```python
from build123d import *

# Parameters (mm, degrees)
BOSS_EXTRUDE1_DEPTH = 13.2
CUT_EXTRUDE1_DEPTH  = 2.2
CUT_EXTRUDE5_DEPTH  = 3.2
CUT_EXTRUDE7_DEPTH  = 47.2


with BuildPart() as part:
    # Sketch1 → Boss-Extrude1 (new body)
    with BuildSketch(Plane(origin=(0, 0, 0), x_dir=(0, 0, -1), z_dir=(1, 0, 0))):
        Polygon((0, 0), (30.22758915, 0), (55.09957656, 33.798540965), (41.306638332, 146.917141225), (-10.793062749, 146.917141225), (-25.237530543, 33.798540965), align=None)
    extrude(amount=BOSS_EXTRUDE1_DEPTH)

    # Sketch2 → Cut-Extrude1 (cut)
    with BuildSketch(Plane(origin=(13.2, 0, 0), x_dir=(0, 0, -1), z_dir=(1, 0, 0))):
        Polygon((28.624161599, 2.054828055), (21.342036292, 2.087122062), (21.778356485, 100.474982686), (42.652153848, 100.428698447), (40.492448974, 94.591340826), (48.720604882, 27.79821975), align=None)
        Polygon((55.09957656, 33.798540965), (46.273401218, 106.183741554), (42.626224982, 94.581878179), (50.828950912, 27.995188239), align=None)
        Polygon((-12.344468939, 94.703766721), (-15.966114176, 106.40555265), (-25.237530543, 33.798540965), (-20.868748173, 27.947791436), align=None)
        Polygon((8.529328424, 100.504360243), (8.529328424, 2.115532151), (1.247131511, 2.115532151), (-18.734951184, 27.947791436), (-10.21067195, 94.703766721), (-12.344468939, 100.550644482), align=None)
        Polygon((-10.793062749, 146.917141225), (-11.605073068, 140.558065069), (0, 140.558065069), (2.885234275, 137.672830794), (15.236290042, 137.672830794), (15.256787792, 146.917141225), align=None)
        Polygon((41.306638332, 146.917141225), (15.256787792, 146.917141225), (15.236290042, 137.672830794), (25.738927324, 137.672830794), (28.624161599, 140.558065069), (42.08202226, 140.558065069), align=None)
    extrude(amount=-CUT_EXTRUDE1_DEPTH, mode=Mode.SUBTRACT)

    # Sketch5 → Cut-Extrude5 (cut)
    with BuildSketch(Plane(origin=(13.2, 0, 0), x_dir=(0, 0, -1), z_dir=(1, 0, 0))):
        Polygon((6.582413404, 94.703766721), (-10.21067195, 94.703766721), (-18.734951184, 27.947791436), (1.247131511, 2.115532151), (6.582413404, 2.115532151), align=None)
        Polygon((49.016878853, 27.881849151), (40.622561704, 94.654291163), (23.829508165, 94.686980269), (23.649277638, 2.098921115), (28.984549423, 2.088535555), align=None)
    extrude(amount=-CUT_EXTRUDE5_DEPTH, mode=Mode.SUBTRACT)

    # Sketch8 → Cut-Extrude7 (cut)
    with BuildSketch(Plane(origin=(10, 0, 0), x_dir=(0, 0, -1), z_dir=(1, 0, 0))):
        Polygon((6.582413404, 94.703766721), (-6.314173101, 90.065077615), (-13.364980543, 27.947791436), (4.888229968, 5.020235463), (6.582413404, 5.020235463), align=None)
        Polygon((25.349112106, 5.000321059), (23.654931879, 5.003618925), (23.829508165, 94.686980269), (36.717040651, 90.023195697), (43.646918386, 27.892302235), align=None)
    extrude(amount=-CUT_EXTRUDE7_DEPTH, mode=Mode.SUBTRACT)


solid = part.part
```
Geometry: final body of the model. Coordinates: model frame, mm. A direction names the side the tool comes from. Give positions to 0.01 mm unless a question says otherwise; leave off trailing zeros. Loops run counter-clockwise (first coordinate to the right, second up) from the corner with the lowest first, then second, coordinate; pieces in that order, holes last. Notation, with made-up numbers: (-34, 75.25) -> (0, 75.25) arc R15 cw to (0, 88.25) -> close; hole circle Ø3 at (72, 63.25). An arc over 180 degrees is marked (long way). Use CSV: the item, a comma, the result in double quotes.
(1) Cut plane A-A (x = 5.75). Output: boundary loops of the cut face in (y, z), plus the area to 3 significant figures.
From the geometry:
outline,"(0, -30.23) -> (33.8, -55.1) -> (146.92, -41.31) -> (146.92, 10.79) -> (33.8, 25.24) -> (0, 0) -> close; hole (5, -25.35) -> (27.89, -43.65) -> (90.02, -36.72) -> (94.69, -23.83) -> (5, -23.65) -> close; hole (5.02, -6.58) -> (94.7, -6.58) -> (90.07, 6.31) -> (27.95, 13.36) -> (5.02, -4.89) -> close"
area,"6,760 mm^2"
(2) Ray query, line 1 along Z through (x, y) = (5.25, 54); line 2 along Z through (x, y) = (8.5, 17.5); line 3 along X through (y, z) = (7, -27). Return the intervals inside material, ascending. Write a range as [from, to].
From the geometry:
line 1,"[-52.64, -40.73], [-23.75, -6.58], [10.41, 22.66]"
line 2,"[-43.11, -35.34], [-23.68, -6.58], [5.05, 13.07]"
line 3,"[0, 10]"
(3) First-contact query: P1, Ø0.7, axis at x = 12, z = 7, coming from the +Y side; P2, Ø0.7, axis at x = 12, z = -16, coming from the +Y side; P3, Ø4.5, axis at y = 140.5, z = -25, coming from the +X side. Flat tips, straight axial feed; report the tip coordinate or a pass-through.
From the geometry:
P1,"y = 140.56"
P2,"y = 137.67"
P3,"x = 11"
(4) Cut plane B-B (y = 46.5). Output: boundary loops of the cut face in (x, z).
From the geometry:
outline,"(0, -53.55) -> (11, -53.55) -> (11, -48.55) -> (13.2, -48.55) -> (13.2, -46.68) -> (10, -46.68) -> (10, -41.57) -> (0, -41.57) -> close; (0, -23.74) -> (11, -23.74) -> (11, -21.54) -> (13.2, -21.54) -> (13.2, -8.53) -> (11, -8.53) -> (11, -6.58) -> (0, -6.58) -> close; (0, 11.26) -> (10, 11.26) -> (10, 16.37) -> (13.2, 16.37) -> (13.2, 18.5) -> (11, 18.5) -> (11, 23.62) -> (0, 23.62) -> close"
(5) Cut plane C-C (y = 80). Output: boundary loops of the cut face in (x, z) (3 decimals), plus the area to 3 significant figures.
From the geometry:
outline,"(0, -49.466) -> (11, -49.466) -> (11, -44.423) -> (13.2, -44.423) -> (13.2, -42.465) -> (10, -42.465) -> (10, -37.835) -> (0, -37.835) -> close; (0, -23.801) -> (11, -23.801) -> (11, -21.688) -> (13.2, -21.688) -> (13.2, -8.529) -> (11, -8.529) -> (11, -6.582) -> (0, -6.582) -> close; (0, 7.457) -> (10, 7.457) -> (10, 12.088) -> (13.2, 12.088) -> (13.2, 14.222) -> (11, 14.222) -> (11, 19.338) -> (0, 19.338) -> close"
area,"477 mm^2"
(6) Access query for faces 1 (the face through (11, 64, 18)), 2 (the face through (12.115, 139.095, -27.161)), 3 (the face through (11.622, 60.858, 14.532)), 4 (the face through (5.07, 59.44, 9.79)). Directions: +Z, -Z, +X, -X, +Y, -Y. A direction counts if a zero-diameter tool reaches every point of the face in a straight line with its end or side. Return the directions, or none.
From the geometry:
face 1,"+Z, +X"
face 2,"+X, +Y"
face 3,"+X"
face 4,"+X, -X"
(7) Pull-direction query (Z, two-part tool) for faces 5 (the face through (12, 2.116, -5)), 6 (the face through (6.51, 17.14, 12.8)), 7 (the face through (6.51, 89.57, -48.3)); classes: released by +Z, released by -Z, zero draft, split by the parting line, or undercut.
From the geometry:
face 5,"undercut"
face 6,"released by +Z"
face 7,"released by -Z"
